Geometry check sheet. Reference: the model listing, model coordinates, mm. A direction names the side the tool comes from. Give positions to 0.01 mm unless a question says otherwise; leave off trailing zeros. Write each loop counter-clockwise with the first axis right and the second up, starting at its lowest first coordinate (ties: lowest second). Pieces come first, ordered by that corner, then holes. Notation, with made-up numbers: (77, -7.75) - (89, -7.75) arc R14 cw to (89, 8.25) - close; hole circle Ø7 at (66, 84.5). An arc over 180 degrees is marked (long way). Use a Markdown table: item, result.
```python
from build123d import *

# Parameters (mm, degrees)
SKETCH_1_W          = 12.5
SKETCH_1_H          = 30
EXTRUDE_1_DEPTH     = 1
SCALE_1_SCALE       = 1.2
FILLET_1_R          = 2
FILLET_2_R          = 3
FILLET_3_R          = 2
CUT_EXTRUDE_1_DEPTH = 0.2


with BuildPart() as part:
    # 草图1 → 凸台-拉伸1 (new body)
    with BuildSketch(Plane(origin=(0, 0, 0), x_dir=(1, 0, 0), z_dir=(0, 1, 0))):
        with Locations((6.25, -15)):
            Rectangle(SKETCH_1_W, SKETCH_1_H)
        Polygon((25, -5), (12.5, 0), (12.5, -30), (25, -25), align=None)
        Polygon((0, -15), (0, -10), (-5, -15), align=None)
        Polygon((0, -20), (0, -15), (-5, -15), align=None)
    extrude(amount=EXTRUDE_1_DEPTH)


with BuildPart() as part_1:
    # 缩放比例1: scaled about (11.271929825, 0.5, 15)
    add(part.part.scale(SCALE_1_SCALE).moved(Location((-2.254385965, -0.1, -3))))

    # 圆角1
    fillet_1_edges = [part_1.edges().sort_by_distance(p)[0] for p in [
        (-8.254385965, 0.5, 15),
    ]]
    fillet(fillet_1_edges, radius=FILLET_1_R)

    # 圆角2
    fillet_2_edges = [part_1.edges().sort_by_distance(p)[0] for p in [
        (-2.254385965, 0.5, -3),
        (12.745614035, 0.5, -3),
        (27.745614035, 0.5, 3),
        (27.745614035, 0.5, 27),
        (12.745614035, 0.5, 33),
        (-2.254385965, 0.5, 33),
    ]]
    fillet(fillet_2_edges, radius=FILLET_2_R)

    # 圆角3
    fillet_3_edges = [part_1.edges().sort_by_distance(p)[0] for p in [
        (-2.254385965, 0.5, 9),
        (-2.254385965, 0.5, 21),
    ]]
    fillet(fillet_3_edges, radius=FILLET_3_R)

    # 草图2 → 切除-拉伸1 (cut)
    with BuildSketch(Plane(origin=(0, 1.1, 0), x_dir=(1, 0, 0), z_dir=(0, 1, 0))):
        Polygon((27.146025588, -15), (12.735189388, -0.589163799), (-1.675646813, -15), (12.735189388, -29.410836201), align=None)
    extrude(amount=-CUT_EXTRUDE_1_DEPTH, mode=Mode.SUBTRACT)


solid = part_1.part
```
1) Mould release check, pull along X, two halves, no side actions. Record for faces 3 (the cylindrical face through (-7.426, 0.508, 14.978)), 4 (the cylindrical face through (27.244, 0.508, 26.63)), 5 (the flat face through (13, 0.9, 15)): pulls with the +X half, pulls with the -X half, needs draft (parallel to the pull), parting line crosses it, or undercut.
Working result:
| item | result |
|---|---|
| face 3 | pulls with the -X half |
| face 4 | pulls with the +X half |
| face 5 | undercut |
2) Depth check by flat-ended pin: P1, Ø0.6, axis at y = 0.5, z = 4.5, coming from the -X side; P2, Ø8.5, axis at x = 13.5, z = 15, coming from the +Y side. Enter the tip coordinate at first touch or a pass-through.
Working result:
| item | result |
|---|---|
| P1 | stops at x = -2.25 |
| P2 | stops at y = 0.9 |
3) Set-up check for faces 1 (the flat face through (-2.254, 0.5, 26)), 2 (the flat face through (19.659, 0.492, -0.235)): record each of +Z, -Z, +X, -X, +Y, -Y from which the full face is reachable in a straight line by a thin tool's end or side.
Working result:
| item | result |
|---|---|
| face 1 | +Z, -X, +Y, -Y |
| face 2 | -Z, +X, +Y, -Y |
4) Section check D-D on z = -1. Record the boundary of the cut face in (x, y).
Working result:
| item | result |
|---|---|
| outline | (-2.08, -0.1) - (17.75, -0.1) - (17.75, 1.1) - (-2.08, 1.1) - close |
5) Section check B-B on z = 4. Record the boundary of the cut face in (x, y), then the cut area to 3 significant figures.
Working result:
| item | result |
|---|---|
| outline | (-2.25, -0.1) - (27.56, -0.1) - (27.56, 1.1) - (16.15, 1.1) - (16.15, 0.9) - (9.32, 0.9) - (9.32, 1.1) - (-2.25, 1.1) - close |
| area | 34.4 mm² |
6) Section check C-C on y = 0.15. Record the boundary of the cut face in (x, z).
Working result:
| item | result |
|---|---|
| outline | (-6.84, 13.59) - (-2.84, 9.59) arc R2 cw to (-2.25, 8.17) - (-2.25, 0) arc R3 ccw to (0.75, -3) - (12.17, -3) arc R3 ccw to (13.28, -2.79) - (25.86, 2.25) arc R3 ccw to (27.75, 5.03) - (27.75, 24.97) arc R3 ccw to (25.86, 27.75) - (13.28, 32.79) arc R3 ccw to (12.17, 33) - (0.75, 33) arc R3 ccw to (-2.25, 30) - (-2.25, 21.83) arc R2 cw to (-2.84, 20.41) - (-6.84, 16.41) arc R2 ccw to start |
7) Section check A-A on x = 5. Record the boundary of the cut face in (y, z), then the cut area to 3 significant figures.
Working result:
| item | result |
|---|---|
| outline | (-0.1, -3) - (1.1, -3) - (1.1, 8.32) - (0.9, 8.32) - (0.9, 21.68) - (1.1, 21.68) - (1.1, 33) - (-0.1, 33) - close |
| area | 40.5 mm² |
8) Material ranges on L1, parallel to Y at x = 11, z = 26; L2, parallel to X at y = 0.1, z = 23.5; L3, parallel to X at y = 0.05, z = 17, recorded low to high. Write a range as from..to.
Working result:
| item | result |
|---|---|
| L1 | y = -0.1..0.9 |
| L2 | x = -2.25..27.75 |
| L3 | x = -6.25..27.75 |
